CAD build for the part. Positions are in the model's coordinates, mm. A direction names the side the tool comes from. Coordinates: 2 decimals unless noted, no trailing zeros. Loops run counter-clockwise (first coordinate to the right, second up) from the corner with the lowest first, then second, coordinate; pieces in that order, holes last. Notation, with made-up numbers: (-19, 19.25) - (-7, 19.25) arc R21 cw to (-7, 43.25) - close; hole circle Ø1 at (83.25, 43.5). An arc over 180 degrees is marked (long way). Put each result on its own line as item: value.
```python
from build123d import *

# Parameters (mm, degrees)
F1_DEPTH = 50
F2_R     = 5
F3_R     = 8.5
F4_DEPTH = 20.001
F5_R     = 6
F6_DEPTH = 25


with BuildPart() as f1:
    # F0 (on Top) → F1 (new body)
    with BuildSketch(Plane.XY):
        with BuildLine():
            ThreePointArc((-20, 0), (0, 20), (20, 0))
            Line((20, 0), (20, -81.932239))
            Line((20, -81.932239), (40, -81.932239))
            Line((40, -81.932239), (40, 38.620689))
            Line((40, 38.620689), (-40, 38.620689))
            Line((-40, 38.620689), (-40, -20.34483))
            Line((-40, -20.34483), (-20, -20.34483))
            Line((-20, -20.34483), (-20, 0))
        make_face()
    extrude(amount=F1_DEPTH)

    # F2
    f2_edges = [f1.edges().sort_by_distance(p)[0] for p in [
        (-40, 38.620689, 25),
        (40, 38.620689, 25),
        (30, -81.932239, 50),
        (30, -81.932239, 0),
    ]]
    fillet(f2_edges, radius=F2_R)

    # F3 (on face) → F4 (cut, through all)
    with BuildSketch(Plane(origin=(20, 0, 0), x_dir=(0, -1, 0), z_dir=(-1, 0, 0))):
        with Locations((38.466119, 37.150957)):
            Circle(F3_R)
        with Locations((38.466119, 14.330863)):
            Circle(F3_R)
    extrude(amount=-F4_DEPTH, mode=Mode.SUBTRACT)

    # F5 (on face) → F6 (cut)
    with BuildSketch(Plane.XZ.offset(20.34483)):
        with Locations((-30, 37.447322)):
            Circle(F5_R)
        with Locations((-30, 16.405419)):
            Circle(F5_R)
    extrude(amount=-F6_DEPTH, mode=Mode.SUBTRACT)


solid = f1.part
```
Q1. Mould opens along X. For faces 4 (the flat face through (-30, 4.655, 16)), 5 (the cylindrical face through (-38.5, 37.19, 25.35)), 6 (the flat face through (-30, -20.345, 25)) say: +X half, -X half, draft (parallel to the pull), parting line (faces both ways), or undercut.
Determined:
face 4: undercut
face 5: -X half
face 6: draft
Q2. Pin check, flat tips, straight feed: pin 1 Ø4 at (y, z) = (-29.5, 8.5) entering from -X; pin 2 Ø6 at (x, z) = (-31, 36.5) entering from -Y; pin 3 Ø16 at (x, z) = (-35, 31) entering from -Y. Stop position of each tip, or through.
Determined:
pin 1: x = 20
pin 2: y = 4.66
pin 3: y = -20.34
Q3. Slice it at D-D, the plane y = 11.5. Give the cut face in (x, z).
Determined:
outline: (-40, 0) - (-16.36, 0) - (-16.36, 50) - (-40, 50) - close; (16.36, 0) - (40, 0) - (40, 50) - (16.36, 50) - close
Q4. Tool access for faces 1 (the flat face through (8, 20, 0)), 2 (the flat face through (-20, -10, 25)), 3 (the flat face through (-30, 4.655, 38)): list every direction of +Z, -Z, +X, -X, +Y, -Y with a clear straight run to the whole face (end or side of a thin tool).
Determined:
face 1: -Z, +X, -X, +Y, -Y
face 2: +Z, -Z, -Y
face 3: -Y
Q5. Slice it at B-B, the plane y = -17. Give the cut face in (x, z), then the cut area to 3 significant figures.
Determined:
outline: (-40, 0) - (-20, 0) - (-20, 50) - (-40, 50) - close; (20, 0) - (40, 0) - (40, 50) - (20, 50) - close; hole circle Ø12 at (-30, 16.41); hole circle Ø12 at (-30, 37.45)
area: 1,770 mm2
Q6. Slice it at A-A, the plane z = 18.5. Give the cut face in (x, y), then the cut area to 3 significant figures.
Determined:
outline: (-40, -20.34) - (-35.62, -20.34) - (-35.62, 4.66) - (-24.38, 4.66) - (-24.38, -20.34) - (-20, -20.34) - (-20, 0) arc R20 cw to (20, 0) - (20, -31.06) - (40, -31.06) - (40, 33.62) arc R5 ccw to (35, 38.62) - (-35, 38.62) arc R5 ccw to (-40, 33.62) - close; (20, -81.93) - (40, -81.93) - (40, -45.87) - (20, -45.87) - close
area: 3,920 mm2
Q7. Slice it at C-C, the plane x = -30. Give the cut face in (y, z), then the cut area to 3 significant figures.
Determined:
outline: (-20.34, 0) - (38.62, 0) - (38.62, 50) - (-20.34, 50) - (-20.34, 43.45) - (4.66, 43.45) - (4.66, 31.45) - (-20.34, 31.45) - (-20.34, 22.41) - (4.66, 22.41) - (4.66, 10.41) - (-20.34, 10.41) - close
area: 2,350 mm2
Q8. Wall check: L1, parallel to X at y = -13.5, z = 16; L2, parallel to X at y = 0.5, z = 33; L3, parallel to Z at x = -30, y = -8. Give the ranges that are in metal, low to high. Write a range as from..to.
Determined:
L1: -40..-35.99, -24.01..-20, 20..40
L2: -40..-34.03, -25.97..-19.99, 19.99..40
L3: 0..10.41, 22.41..31.45, 43.45..50
